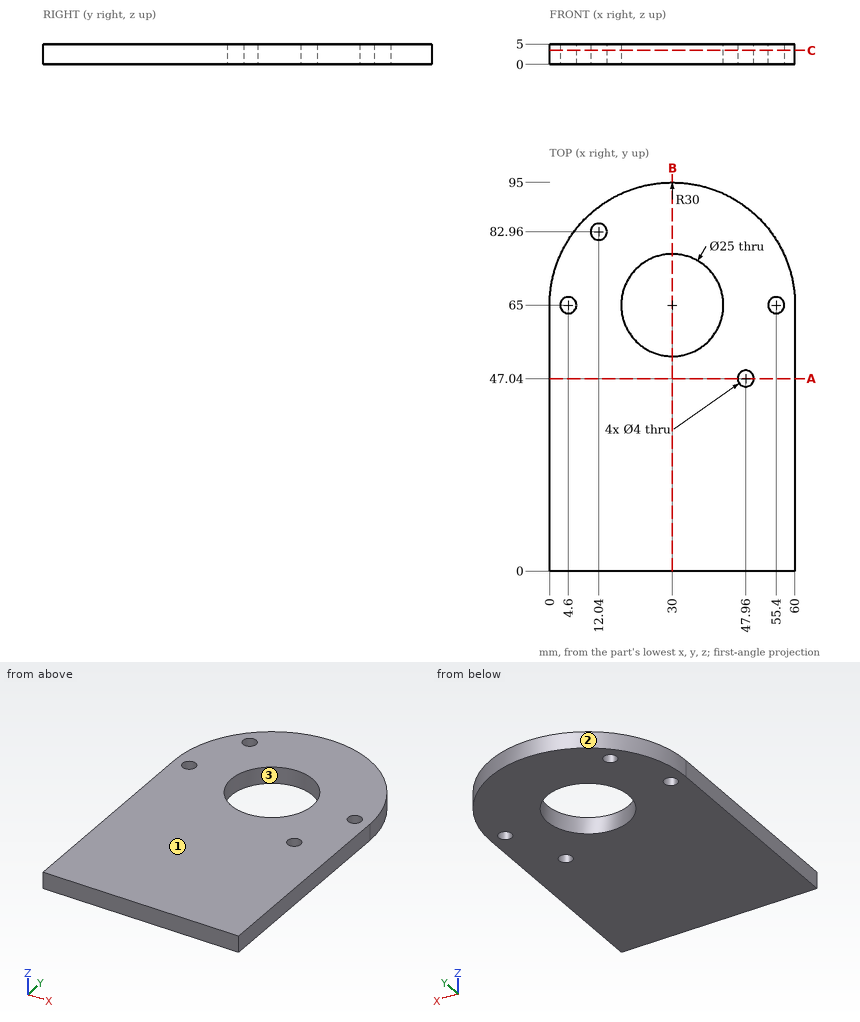
Study the drawing (mm; zero at the part's minimum x, y, z) and answer. Give positions to 0.01 mm unless a question says otherwise; leave off trailing zeros. Loops run counter-clockwise (first coordinate to the right, second up) from the corner with the lowest first, then second, coordinate; pieces in that order, holes last. Notation, with made-up numbers: M 18,-25 L 58,-25 A4 cw 58,-19 Z; hole C 5.25,32 d10. An arc over 180 degrees is marked long. Answer as CSV lines item,"result".
Item 1: The part is cut by section C-C (z = 3.45). Give the vertices of the cut face in (x, y).
Values follow:
outline,"M 0,0 L 60,0 L 60,65 A30 ccw 0,65 Z; hole C 4.6,65 d4; hole C 12.04,82.96 d4; hole C 30,65 d25; hole C 47.96,47.04 d4; hole C 55.4,65 d4"
Item 2: The part is cut by section A-A (y = 47.04). Give the vertices of the cut face in (x, z), and give its area (3 significant figures).
Values follow:
outline,"M 0,0 L 45.96,0 L 45.96,5 L 0,5 Z; M 49.96,0 L 60,0 L 60,5 L 49.96,5 Z"
area,"280 mm^2"
Item 3: Straight lines are drawn through the part: line 1 along Y through (x, z) = (55.4, 1.4); line 2 along Y through (x, z) = (30.5, 0.25); line 3 along X through (y, z) = (46.5, 1.6). For each, find the intervals that lie inside material, in ascending order. Write a range as [from, to].
Values follow:
line 1,"y = [0, 63], [67, 80.96]"
line 2,"y = [0, 52.51], [77.49, 95]"
line 3,"x = [0, 46.03], [49.89, 60]"
Item 4: The mould has two halves that part along X. Classify the marked faces 1, 2 and 3: released by +X, released by -X, zero draft, split by the parting line, or undercut.
Values follow:
face 1,"zero draft"
face 2,"split by the parting line"
face 3,"undercut"
Item 5: The part is cut by section B-B (x = 30). Give the vertices of the cut face in (y, z), and give its area (3 significant figures).
Values follow:
outline,"M 0,0 L 52.5,0 L 52.5,5 L 0,5 Z; M 77.5,0 L 95,0 L 95,5 L 77.5,5 Z"
area,"350 mm^2"
Item 6: Given pin 1 Ø3 at (x, y) = (41.5, 43) entering from -Z, flat-ended and moving along its own axis, determine where the tip first touches the part or whether it passes through.
Values follow:
pin 1,"stops at z = 0"
